Work out the finished part from the listing and answer in its coordinate system (mm). A direction names the side the tool comes from. Round coordinates to 2 decimals unless told otherwise and drop trailing zeros. Write each loop counter-clockwise with the first axis right and the second up, starting at its lowest first coordinate (ties: lowest second). Pieces come first, ordered by that corner, then holes. Notation, with made-up numbers: (21.25, 64) - (31.25, 64) arc R30 cw to (31.25, 98) - close; hole circle Ø6 at (-7, -14). An arc over 180 degrees is marked (long way). Answer as a JSON object with one key per item and string values.
```python
from build123d import *

# Parameters (mm, degrees)
SKIZZE1_W                       = 25
SKIZZE1_H                       = 12
SKIZZE1_R                       = 2.75
AUFSATZ_LINEAR_AUSTRAGEN1_DEPTH = 6
SKIZZE2_R                       = 2.75
SKIZZE2_W                       = 12.5
SKIZZE2_H                       = 3
SCHNITT_LINEAR_AUSTRAGEN1_DEPTH = 13
SCHNITT_LINEAR_AUSTRAGEN2_REACH = 27
SKIZZE3_R                       = 1.25


with BuildPart() as part:
    # Skizze1 → Aufsatz-Linear austragen1 (new body, symmetric)
    with BuildSketch(Plane.XY):
        Rectangle(SKIZZE1_W, SKIZZE1_H)
        with Locations((-6.25, 0)):
            Circle(SKIZZE1_R, mode=Mode.SUBTRACT)
    extrude(amount=AUFSATZ_LINEAR_AUSTRAGEN1_DEPTH, both=True)

    # Skizze2 → Schnitt-Linear austragen1 (cut, through all)
    with BuildSketch(Plane(origin=(0, 6, 0), x_dir=(1, 0, 0), z_dir=(0, 1, 0))):
        with Locations((6.25, 0)):
            Circle(SKIZZE2_R)
        with Locations((-6.25, 4.5)):
            Rectangle(SKIZZE2_W, SKIZZE2_H)
        with Locations((-6.25, -4.5)):
            Rectangle(SKIZZE2_W, SKIZZE2_H)
    extrude(amount=-SCHNITT_LINEAR_AUSTRAGEN1_DEPTH, mode=Mode.SUBTRACT)

    # Skizze3 → Schnitt-Linear austragen2 (cut, up to next)
    with BuildSketch(Plane(origin=(12.5, 0, 0), x_dir=(0, 0, -1), z_dir=(1, 0, 0)), mode=Mode.PRIVATE) as schnitt_linear_austragen2_sk1:
        Circle(SKIZZE3_R)
    schnitt_linear_austragen2_tool1 = extrude(schnitt_linear_austragen2_sk1.sketch, amount=-SCHNITT_LINEAR_AUSTRAGEN2_REACH, mode=Mode.PRIVATE) & part.part
    add(schnitt_linear_austragen2_tool1.solids().sort_by_distance((12.5, 0, 0))[0], mode=Mode.SUBTRACT)


solid = part.part
```
Item 1: A cutting plane is placed at D-D (z = -2.25). Write down the section's boundary in (x, y).
Results found:
{"outline": "(-12.5, -6) - (4.67, -6) - (4.67, 6) - (-12.5, 6) - close; (7.83, -6) - (12.5, -6) - (12.5, 6) - (7.83, 6) - close; hole circle Ø5.5 at (-6.25, 0)"}
Item 2: Consider line 1 along Y through (x, z) = (-6.25, -1.35); line 2 along Y through (x, z) = (9.8, 0). Determine where each line is inside the solid, lowest interval first.
Results found:
{"line 1": "-6 to -2.75, 2.75 to 6", "line 2": "-6 to -1.25, 1.25 to 6"}
Item 3: For faces 1 (the flat face through (0, 0, 5)), 2 (the flat face through (0, -6, 0)), 3 (the flat face through (-6, 3, -3)), determine the directions among +Z, -Z, +X, -X, +Y, -Y from which every point of the face is accessible in a straight line to the end or side of a thin tool.
Results found:
{"face 1": "+Z, -X, +Y, -Y", "face 2": "+Z, -Z, +X, -X, -Y", "face 3": "-Z, -X, +Y, -Y"}
Item 4: A cutting plane is placed at C-C (x = 6.25). Write down the section's boundary in (y, z).
Results found:
{"outline": "(-6, -6) - (6, -6) - (6, -2.75) - (-6, -2.75) - close; (-6, 2.75) - (6, 2.75) - (6, 6) - (-6, 6) - close"}
Item 5: Determine the mould class of faces 4 (the flat face through (-6, 3, 3)), 5 (the cylindrical face through (10.63, 1.24, 0.16)), 6 (the flat face through (12.5, -0.1, 1.4)) for opening direction Z: pulls with the +Z half, pulls with the -Z half, needs draft (parallel to the pull), parting line crosses it, or undercut.
Results found:
{"face 4": "pulls with the +Z half", "face 5": "undercut", "face 6": "needs draft"}
Item 6: A cutting plane is placed at A-A (z = 0). Write down the section's boundary in (x, y).
Results found:
{"outline": "(-12.5, -6) - (3.5, -6) - (3.5, 6) - (-12.5, 6) - close; (9, -6) - (12.5, -6) - (12.5, -1.25) - (9, -1.25) - close; (9, 1.25) - (12.5, 1.25) - (12.5, 6) - (9, 6) - close; hole circle Ø5.5 at (-6.25, 0)"}
Item 7: Each of these flat-tipped pins is pushed along its axis until it touches: P1, Ø1.5, axis at y = 0, z = -5, coming from the -X side; P2, Ø6, axis at x = -8.5, y = -2, coming from the +Z side. Where does it stop, or does it pass through?
Results found:
{"P1": "x = 0", "P2": "z = 3"}
Item 8: A cutting plane is placed at B-B (y = -1.75). Write down the section's boundary in (x, z), and give its area (3 significant figures).
Results found:
{"outline": "(-12.5, -3) - (-8.37, -3) - (-8.37, 3) - (-12.5, 3) - close; (-4.13, -3) - (0, -3) - (0, -6) - (12.5, -6) - (12.5, 6) - (0, 6) - (0, 3) - (-4.13, 3) - close; hole circle Ø5.5 at (6.25, 0)", "area": "176 mm²"}
